Can you work these out from the model? Positions are in its coordinate system, mm. A direction names the side the tool comes from. Coordinates: 2 decimals unless noted, no trailing zeros. Order: outer loops, then holes, each group sorted by start corner. A loop starts at its lowest first (then second) coordinate and runs counter-clockwise, first axis right, second up. Notation, with made-up numbers: (-12, -29) - (6, -29) arc R16 cw to (6, -18) - close; hole circle Ø5 at (-10.75, 46.25). An arc over 180 degrees is marked (long way). Return JSON: item names as keys, results as strings. Group by question number.
1) For pin 1 Ø0.5 at (y, z) = (-1, 3) entering from -X; pin 2 Ø1.5 at (x, z) = (8.5, 3.5) entering from +Y; pin 3 Ø3 at (x, z) = (3.5, 1.5) entering from +Y; pin 4 Ø1.2 at (x, y) = (9.65, 1.5) entering from +Z, each with a flat end and sliding along its axis, tell me the tip position at first contact or that it passes through.
2) Imagine slicing it at A-A (y = -0.25). Write out the boundary of the cut face in (x, z) (3 decimals), and give its area (3 significant figures).
3) If I drill on line 1 along X through (y, z) = (1.5, 1.3); line 2 along X through (y, z) = (-2.5, 2.8); line 3 along Y through (x, z) = (9.65, 2.25), over which ranges is the centre line in solid material (lowest first)?
4) If we mould it in two halves opening along Y, with no side actions, what happens to faces 6 (the face through (11.5, -1.3, 3.105)), 7 (the face through (4.126, 1.717, 2.761)), 8 (the face through (10.626, 1.717, 2.761)), 9 (the face through (6.974, 8.174, 2.825))? For each: pulls with the +Y half, pulls with the -Y half, needs draft (parallel to the pull), parting line crosses it, or undercut.
5) Imagine slicing it at D-D (x = 6.5). Write out the boundary of the cut face in (y, z).
6) Which directions (+Z, -Z, +X, -X, +Y, -Y) give clear straight access to the entire face, cutting with the end or side of a thin tool? Please do faces 1 (the face through (7, 8, 4.6)), 2 (the face through (7, 8, 1)), 3 (the face through (11.5, -1.3, 2.505)), 4 (the face through (7.023, 7.675, 2.825)), 5 (the face through (12.8, 3, 3)).
7) Imagine slicing it at C-C (x = 9). Write out the boundary of the cut face in (y, z).
8) Imagine slicing it at B-B (z = 1.75). Give the number of separate pieces and of enclosed holes in the cut face, and give its area (3 significant figures).
Autodesk Inventor part; units mm, degrees
ref_plane "YZ Plane" through (0, 0, 0) normal (1, 0, 0) x (0, 1, 0)
ref_plane "XZ Plane" through (0, 0, 0) normal (0, 1, 0) x (-1, 0, 0)
ref_plane "XY Plane" through (0, 0, 0) normal (0, 0, 1) x (1, 0, 0)
sketch "Sketch1" plane through (0, 0, 0) normal (0, 0, 1) x (1, 0, 0)
  line L0 (0, 0) -> (12.8, 0)
  line L1 (12.8, 0) -> (12.8, 6.5)
  line L2 (12.8, 6.5) -> (0, 6.5)
  line L3 (0, 6.5) -> (0, 0)
  dimension "d0" = 12.8
  dimension "d1" = 6.5
extrude "Extrusion1" add sketch "Sketch1" along normal blind 5.6
sketch "Sketch2" plane through (0, 0, 5.6) normal (0, 0, 1) x (1, 0, 0)
  line L0 (0, 0) -> (0, 6.5)
  line L1 (12.8, 0) -> (0, 0)
  point P0 (3.15, 1.5)
  point P1 (9.65, 1.5)
  dimension "d4" = 6.5
  dimension "d5" = 3.15
  dimension "d6" = 1.5
hole "Hole1" at (3.15, 1.5, 5.6) at (9.65, 1.5, 5.6) direction (0, 0, -1) diameter 2 end through all
sketch "Sketch3" plane through (0, 0, 5.6) normal (0, 0, 1) x (1, 0, 0)
  line L0 (12.8, 0) -> (0, 0)
  line L1 (0, 0) -> (2.225, 0)
  line L2 (2.225, 0) -> (2.225, 0)
  line L3 (1.725, 0.5) -> (0, 0.5)
  line L4 (0, 0.5) -> (0, 0)
  line L5 (4.525, 0.5) -> (8.275, 0.5)
  line L6 (8.775, 0) -> (8.775, 0)
  line L7 (8.775, 0) -> (4.025, 0)
  line L8 (4.025, 0) -> (4.025, 0)
  line L9 (11.075, 0.5) -> (12.8, 0.5)
  line L10 (12.8, 0.5) -> (12.8, 0)
  line L11 (12.8, 0) -> (10.575, 0)
  line L12 (10.575, 0) -> (10.575, 0)
  line L13 (1.725, 0.5) -> (2.225, 0)
  line L14 (4.525, 0.5) -> (4.025, 0)
  line L15 (8.275, 0.5) -> (8.775, 0)
  line L16 (11.075, 0.5) -> (10.575, 0)
  point P0 (2.225, 0.5)
  point P1 (4.025, 0.5)
  point P2 (8.775, 0.5)
  point P3 (10.575, 0.5)
  dimension "d14" = 0.5
  dimension "d17" = 2.225
  dimension "d18" = 2.225
  dimension "d19" = 0.5
  dimension "d20" = 0.5
  dimension "d21" = 0.5
  dimension "d22" = 0.5
  dimension "d23" = 0.5
  dimension "d24" = 0.5
  dimension "d25" = 0.5
  dimension "d26" = 0.5
  dimension "d49" = 1.8
  dimension "d50" = 1.8
extrude "Extrusion2" cut sketch "Sketch3" against normal through all
sketch "Sketch4" plane through (0, 6.5, 0) normal (0, 1, 0) x (1, 0, 0)
  line L0 (12.8, 0) -> (0, 0)
  line L1 (0, 0) -> (0, -5.6)
  line L2 (0.5, -1) -> (1, -1)
  line L3 (1, -1) -> (1, -4.6)
  line L4 (1, -4.6) -> (0.5, -4.6)
  line L5 (0.5, -4.6) -> (0.5, -1)
  dimension "d29" = 3.6
  dimension "d30" = 1
  dimension "d31" = 0.5
  dimension "d32" = 0.5
extrude "Extrusion3" add sketch "Sketch4" along normal blind 0.5
sketch "Sketch5" plane through (0.5, 6.5, 4.6) normal (0, 0, 1) x (1, 0, 0)
  line L0 (0, 0.5) -> (12.6283, 2.79)
  line L1 (0.0892, 0.008) -> (12.7175, 2.298)
  line L2 (12.6283, 2.79) -> (12.7175, 2.298)
  line L3 (0, 0.5) -> (0.0892, 0.008)
  dimension "d35" = 0.5
extrude "Extrusion4" add sketch "Sketch5" against normal blind 3.6
fillet "Fillet1" radius 0.6 1 edges at (0.5, 7, 2.8)
sketch "Sketch6" plane through (4.525, 0.5, 5.6) normal (0, -1, 0) x (1, 0, 0)
  line L0 (1.475, -2.5) -> (2.275, -2.5)
  line L1 (2.275, -2.5) -> (2.275, -3.1)
  line L2 (2.275, -3.1) -> (1.475, -3.1)
  line L3 (1.475, -3.1) -> (1.475, -2.5)
  line L4 (-3.605, -2.495) -> (-2.805, -2.495)
  line L5 (-2.805, -2.495) -> (-2.805, -3.095)
  line L6 (-2.805, -3.095) -> (-3.605, -3.095)
  line L7 (-3.605, -3.095) -> (-3.605, -2.495)
  line L8 (6.555, -2.495) -> (7.355, -2.495)
  line L9 (7.355, -2.495) -> (7.355, -3.095)
  line L10 (7.355, -3.095) -> (6.555, -3.095)
  line L11 (6.555, -3.095) -> (6.555, -2.495)
  line L12 (-4.525, -5.6) -> (-4.525, 0)
  line L13 (0, 0) -> (3.75, 0)
  dimension "d39" = 0.6
  dimension "d40" = 0.8
  dimension "d41" = 0.8
  dimension "d42" = 0.8
  dimension "d43" = 4.28
  dimension "d44" = 4.28
  dimension "d45" = 0.92
  dimension "d48" = 2.5
extrude "Extrusion5" add sketch "Sketch6" along normal blind 3.6
properties part number "switch"
Calculated:
{
 "1": {"pin 1": "x = 0.92", "pin 2": "y = 8.59", "pin 3": "y = 7.82", "pin 4": "through"},
 "2": {"outline": "(0.92, 2.505) - (1.72, 2.505) - (1.72, 3.105) - (0.92, 3.105) - close; (6, 2.5) - (6.8, 2.5) - (6.8, 3.1) - (6, 3.1) - close; (11.08, 2.505) - (11.88, 2.505) - (11.88, 3.105) - (11.08, 3.105) - close", "area": "1.44 mm2"},
 "3": {"line 1": "0 to 2.15, 4.15 to 8.65, 10.65 to 12.8", "line 2": "0.92 to 1.72, 6 to 6.8, 11.08 to 11.88", "line 3": "0 to 0.5, 2.5 to 6.5, 8.15 to 8.66"},
 "4": {"face 6": "needs draft", "face 7": "undercut", "face 8": "undercut", "face 9": "pulls with the +Y half"},
 "5": {"outline": "(-3.1, 2.5) - (0.5, 2.5) - (0.5, 0) - (6.5, 0) - (6.5, 5.6) - (0.5, 5.6) - (0.5, 3.1) - (-3.1, 3.1) - close; (7.58, 1) - (8.09, 1) - (8.09, 4.6) - (7.58, 4.6) - close"},
 "6": {"face 1": "+Z, +X, -X, +Y", "face 2": "-Z, +X, -X, +Y", "face 3": "-Z, +X, -Y", "face 4": "+Z, -Z, +X", "face 5": "+Z, -Z, +X, -Y"},
 "7": {"outline": "(0, 0) - (0.74, 0) - (0.74, 5.6) - (0, 5.6) - close; (2.26, 0) - (6.5, 0) - (6.5, 5.6) - (2.26, 5.6) - close; (8.03, 1) - (8.54, 1) - (8.54, 4.6) - (8.03, 4.6) - close"},
 "8": {"separate pieces": "1", "enclosed holes": "2", "area": "79.2 mm2"}
}
